Design review of the part built by this model. Coordinates are the model's own, in mm. Coordinates: 2 decimals unless noted, no trailing zeros. Write each loop counter-clockwise with the first axis right and the second up, starting at its lowest first coordinate (ties: lowest second). Pieces come first, ordered by that corner, then holes.
Q1. Add section C-C, the plane x = 0. Give the boundary of the cut face in (y, z), plus the area to 3 significant figures.
Q2. Add section A-A, the plane x = -107. Give the boundary of the cut face in (y, z), plus the area to 3 significant figures.
Q3. Clearance check with flat-ended pins moving along their axes: pin 1 Ø3 at (x, z) = (-79, 3) entering from -Y; pin 2 Ø1.2 at (x, z) = (-146, 3) entering from +Y. State where each tip first meets the part, or that it passes through.
Q4. Add section D-D, the plane z = 3. Give the number of separate pieces and of enclosed holes in the cut face, plus the area to 3 significant figures.
Q5. To check wall thickness, follow probe 1 along Y at (x, z) = (-137, 2.75); probe 2 along X at (y, z) = (50.75, 3); probe 3 along Y at (x, z) = (-67, 1.2). State the ranges of each line that lie inside material, in increasing order.
Q6. Add section B-B, the plane y = 0. Give the boundary of the cut face in (x, z).
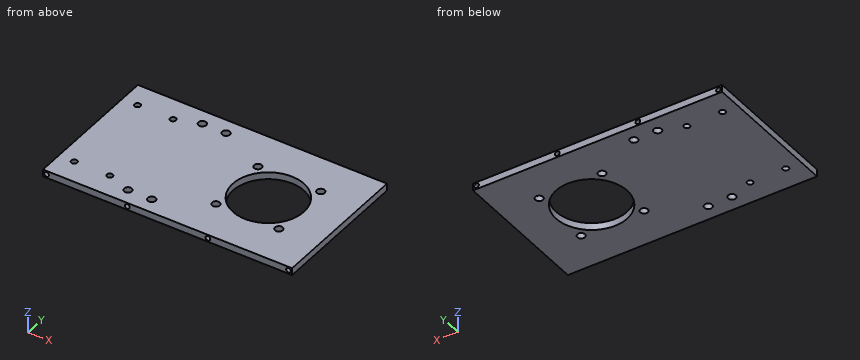
from build123d import *

# Parameters (mm, degrees)
SKETCH_1_W          = 210
SKETCH_1_H          = 120
SKETCH_1_R          = 3.25
SKETCH_1_R_2        = 30
EXTRUDE_1_DEPTH     = 6
SKETCH_2_R          = 2.5
CUT_EXTRUDE_1_DEPTH = 10
SKETCH_3_R          = 2
CUT_EXTRUDE_2_DEPTH = 20
SKETCH_4_R          = 3.3
CUT_EXTRUDE_3_DEPTH = 10


with BuildPart() as part:
    # 草图1 → 凸台-拉伸1 (new body)
    with BuildSketch(Plane.XY):
        with Locations((-45, 0)):
            Rectangle(SKETCH_1_W, SKETCH_1_H)
        with Locations((26.516504294, 26.516504294)):
            Circle(SKETCH_1_R, mode=Mode.SUBTRACT)
        with Locations((26.516504294, -26.516504294)):
            Circle(SKETCH_1_R, mode=Mode.SUBTRACT)
        with Locations((-26.516504294, -26.516504294)):
            Circle(SKETCH_1_R, mode=Mode.SUBTRACT)
        with Locations((-26.516504294, 26.516504294)):
            Circle(SKETCH_1_R, mode=Mode.SUBTRACT)
        Circle(SKETCH_1_R_2, mode=Mode.SUBTRACT)
    extrude(amount=EXTRUDE_1_DEPTH)

    # 草图2 → 切除-拉伸1 (cut)
    with BuildSketch(Plane.XY.offset(6)):
        with Locations((-137, 40)):
            Circle(SKETCH_2_R)
        with Locations((-107, 40)):
            Circle(SKETCH_2_R)
        with Locations((-107, -40)):
            Circle(SKETCH_2_R)
        with Locations((-137, -40)):
            Circle(SKETCH_2_R)
    extrude(amount=-CUT_EXTRUDE_1_DEPTH, mode=Mode.SUBTRACT)

    # 草图3 → 切除-拉伸2 (cut)
    with BuildSketch(Plane(origin=(0, -60, 0), x_dir=(-1, 0, 0), z_dir=(0, -1, 0))):
        with Locations((-57, -3)):
            Circle(SKETCH_3_R)
        with Locations((11, -3)):
            Circle(SKETCH_3_R)
        with Locations((79, -3)):
            Circle(SKETCH_3_R)
        with Locations((147, -3)):
            Circle(SKETCH_3_R)
    cut_extrude_2 = extrude(amount=-CUT_EXTRUDE_2_DEPTH, mode=Mode.SUBTRACT)

    # 镜向3: 切除-拉伸2 across plane
    add(cut_extrude_2.mirror(Plane(origin=(0, 0, 0), x_dir=(0, 0, 1), z_dir=(0, -1, 0))), mode=Mode.SUBTRACT)

    # 草图4 → 切除-拉伸3 (cut)
    with BuildSketch(Plane.XY.offset(6)):
        with Locations((-87, 47)):
            Circle(SKETCH_4_R)
        with Locations((-67, 47)):
            Circle(SKETCH_4_R)
        with Locations((-67, -47)):
            Circle(SKETCH_4_R)
        with Locations((-87, -47)):
            Circle(SKETCH_4_R)
    extrude(amount=-CUT_EXTRUDE_3_DEPTH, mode=Mode.SUBTRACT)


solid = part.part
Here are the results:
1. outline: (-60, 0) - (-30, 0) - (-30, 6) - (-60, 6) - close; (30, 0) - (60, 0) - (60, 6) - (30, 6) - close
1. area: 360 mm2
2. outline: (-60, 0) - (-42.5, 0) - (-42.5, 6) - (-60, 6) - close; (-37.5, 0) - (37.5, 0) - (37.5, 6) - (-37.5, 6) - close; (42.5, 0) - (60, 0) - (60, 6) - (42.5, 6) - close
2. area: 660 mm2
3. pin 1: stops at y = -40
3. pin 2: stops at y = 40
4. separate pieces: 1
4. enclosed holes: 13
4. area: 21,400 mm2
5. probe 1: y = -60 to -42.5, -37.5 to 37.5, 42.5 to 60
5. probe 2: x = -150 to -149, -145 to -81, -77 to -13, -9 to 55, 59 to 60
5. probe 3: y = -60 to -50.3, -43.7 to 43.7, 50.3 to 60
6. outline: (-150, 0) - (-30, 0) - (-30, 6) - (-150, 6) - close; (30, 0) - (60, 0) - (60, 6) - (30, 6) - close
